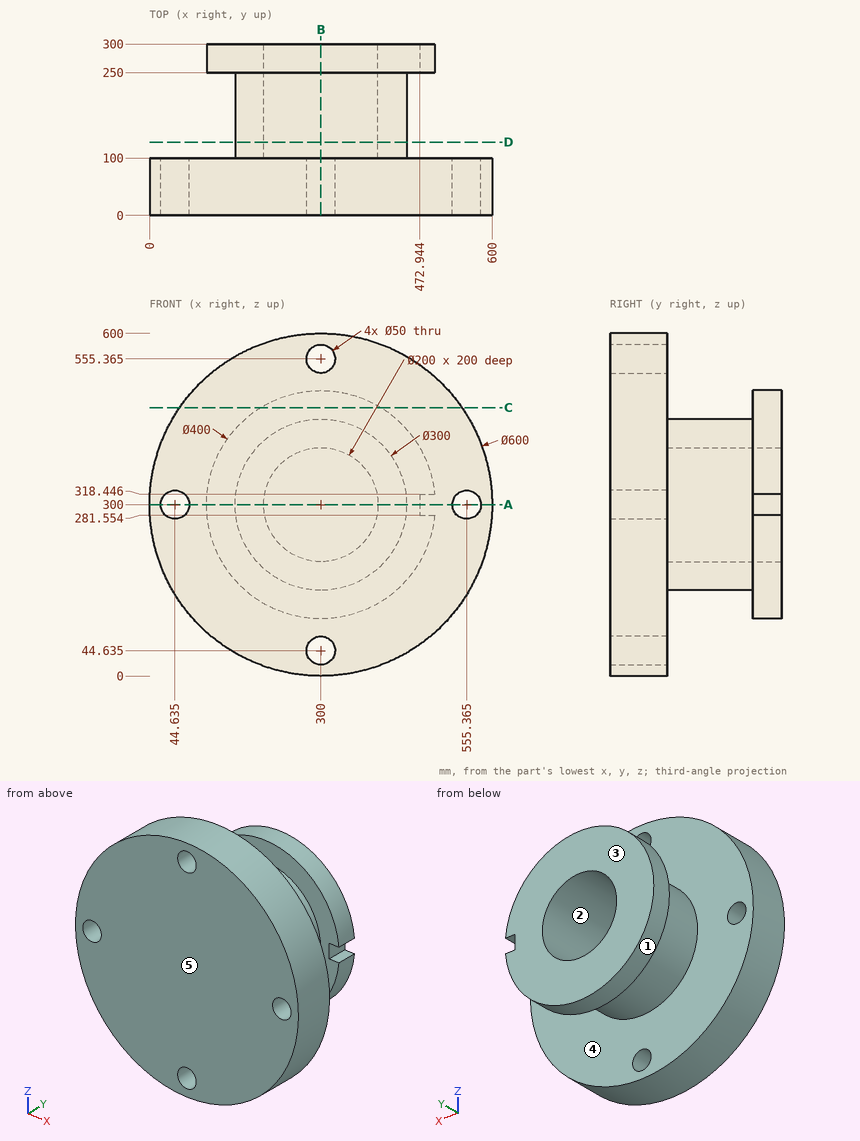
Verification items for this drawing (mm, ordinates from the low corner). A direction names the side the tool comes from. Coordinates: 2 decimals unless noted, no trailing zeros. Write each loop counter-clockwise with the first axis right and the second up, starting at its lowest first coordinate (ties: lowest second). Pieces come first, ordered by that corner, then holes. Notation, with made-up numbers: (14.5, 50) -> (62.5, 50) arc R29 cw to (62.5, 81) -> close; hole circle Ø11 at (-12, 43). An arc over 180 degrees is marked (long way). One line per item, written item: value. Start each with the question number.
Q1. Thickness scan on L1, parallel to Y at x = 349, z = 455.5; L2, parallel to Z at x = 309.5, y = 81.5; L3, parallel to X at y = 214, z = 337 (1 decimal). Record the ranges inside material, lowest first. Write a range as from..to.
Q2. Cross-section at B-B on x = 300. Enter the section's corners in (y, z) (1 decimal).
Q3. Cross-section at C-C on z = 470. Enter the section's corners in (x, y) (1 decimal).
Q4. Access from +Z, -Z, +X, -X, +Y, -Y to the whole of each face (thin tool, end or side, straight path). Record for the marked faces 4 and 5.
Q5. Mould release check, pull along X, two halves, no side actions. Record for the marked faces 1, 2 and 3: pulls with the +X half, pulls with the -X half, needs draft (parallel to the pull), parting line crosses it, or undercut.
Q6. Cross-section at A-A on z = 300. Enter the section's corners in (x, y) (1 decimal).
Q7. Cross-section at D-D on y = 128. Enter the section's corners in (x, z), and give its area (3 significant figures).
Q8. Go/stop test with flat-tipped pins: P1, Ø18.5, axis at y = 287, z = 298.5, coming from the +X side; P2, Ø3, axis at x = 521.5, z = 481, coming from the +Y side; P3, Ø1, axis at y = 34, z = 66, coming from the -X side (1 decimal). Record where each tip stops, or that it passes through.
Checked values:
1. L1: y = 0..100, 250..300
1. L2: z = 0.15..21.51, 67.76..532.24, 578.49..599.85
1. L3: x = 154.6..207.1, 392.9..445.4
2. outline: (0, 0) -> (100, 0) -> (100, 19.6) -> (0, 19.6) -> close; (0, 69.6) -> (100, 69.6) -> (100, 150) -> (250, 150) -> (250, 100) -> (300, 100) -> (300, 200) -> (100, 200) -> (100, 400) -> (300, 400) -> (300, 500) -> (250, 500) -> (250, 450) -> (100, 450) -> (100, 530.4) -> (0, 530.4) -> close; (0, 580.4) -> (100, 580.4) -> (100, 600) -> (0, 600) -> close
3. outline: (52.8, 0) -> (547.2, 0) -> (547.2, 100) -> (52.8, 100) -> close; (194.6, 250) -> (405.4, 250) -> (405.4, 300) -> (194.6, 300) -> close
4. face 4: none
4. face 5: +Z, -Z, +X, -X, -Y
5. face 1: parting line crosses it
5. face 2: undercut
5. face 3: needs draft
6. outline: (0, 0) -> (19.6, 0) -> (19.6, 100) -> (0, 100) -> close; (69.6, 0) -> (530.4, 0) -> (530.4, 100) -> (450, 100) -> (450, 250) -> (472.9, 250) -> (472.9, 300) -> (400, 300) -> (400, 100) -> (200, 100) -> (200, 300) -> (100, 300) -> (100, 250) -> (150, 250) -> (150, 100) -> (69.6, 100) -> close; (580.4, 0) -> (600, 0) -> (600, 100) -> (580.4, 100) -> close
7. outline: circle Ø300 at (300, 300); hole circle Ø200 at (300, 300)
7. area: 39,300 mm²
8. P1: stops at x = 472.94
8. P2: stops at y = 100
8. P3: stops at x = 111.6
